Source: CAD feature listing. Evaluate the final solid. Frame: model axes, mm. A direction names the side the tool comes from. Give positions to 0.01 mm unless a question says otherwise; leave off trailing zeros. Write each loop counter-clockwise with the first axis right and the second up, starting at its lowest first coordinate (ties: lowest second). Pieces come first, ordered by that corner, then holes. Notation, with made-up numbers: (17, 82.25) -> (75, 82.25) arc R29 ccw to (75, 114.25) -> close; hole circle Ø9 at (-8.5, -15.5). An arc over 180 degrees is marked (long way). Write item = value, one per line.
from build123d import *

# Parameters (mm, degrees)
BOSS_EXTRUDE1_DEPTH = 3.5814
SKETCH2_W           = 30
SKETCH2_H           = 4
BOSS_EXTRUDE2_DEPTH = 10
SKETCH3_R           = 1.5
CUT_EXTRUDE1_DEPTH  = 4


with BuildPart() as part:
    # Sketch1 → Boss-Extrude1 (new body)
    with BuildSketch(Plane(origin=(0, 0, 0), x_dir=(1, 0, 0), z_dir=(0, 1, 0))):
        Polygon((-15, -10.05), (15, -10.05), (15, -2.05), (1.7907, -2.05), (1.7907, 2.05), (9.398, 2.05), (1.7907, 7.13), (-1.7907, 7.13), (-9.398, 2.05), (-1.7907, 2.05), (-1.7907, -2.05), (-15, -2.05), align=None)
    extrude(amount=BOSS_EXTRUDE1_DEPTH)

    # Sketch2 → Boss-Extrude2 (add)
    with BuildSketch(Plane(origin=(0, 3.5814, 0), x_dir=(1, 0, 0), z_dir=(0, 1, 0))):
        with Locations((0, -8.05)):
            Rectangle(SKETCH2_W, SKETCH2_H)
    extrude(amount=BOSS_EXTRUDE2_DEPTH)

    # Sketch3 → Cut-Extrude1 (cut)
    with BuildSketch(Plane.XY.offset(10.05)):
        with Locations((-11.65, 6.7907)):
            Circle(SKETCH3_R)
        with Locations((11.65, 6.7907)):
            Circle(SKETCH3_R)
    extrude(amount=-CUT_EXTRUDE1_DEPTH, mode=Mode.SUBTRACT)


solid = part.part
1) Contact query for flat-ended pins moving along their axis: pin 1 (1 mm diameter, centred on x = 10, y = 5, fed in from -Z); pin 2 (1.8 mm diameter, centred on x = -9.5, y = 2, fed in from -Z); pin 3 (10 mm diameter, centred on x = 11, z = -4.5, fed in from +Y). Output: stop coordinate, or through.
Computed:
pin_1 = 6.05
pin_2 = -2.58
pin_3 = 3.58
2) Cut plane B-B (y = 7.25). Return the cut outline in (x, z).
Computed:
outline = (-15, 6.05) -> (-13.08, 6.05) -> (-13.08, 10.05) -> (-15, 10.05) -> close; (-10.22, 6.05) -> (10.22, 6.05) -> (10.22, 10.05) -> (-10.22, 10.05) -> close; (13.08, 6.05) -> (15, 6.05) -> (15, 10.05) -> (13.08, 10.05) -> close
3) Cut plane D-D (z = 9.25). Return the cut outline in (x, y).
Computed:
outline = (-15, 0) -> (15, 0) -> (15, 13.58) -> (-15, 13.58) -> close; hole circle Ø3 at (-11.65, 6.79); hole circle Ø3 at (11.65, 6.79)
4) Cut plane C-C (y = 2.5). Return the cut outline in (x, z), then the cut area to 3 significant figures.
Computed:
outline = (-15, 2.05) -> (-1.79, 2.05) -> (-1.79, -2.05) -> (-9.4, -2.05) -> (-1.79, -7.13) -> (1.79, -7.13) -> (9.4, -2.05) -> (1.79, -2.05) -> (1.79, 2.05) -> (15, 2.05) -> (15, 10.05) -> (-15, 10.05) -> close
area = 312 mm²
5) Cut plane A-A (x = -11.65). Return the cut outline in (y, z), then the cut area to 3 significant figures.
Computed:
outline = (0, 2.05) -> (3.58, 2.05) -> (3.58, 6.05) -> (5.29, 6.05) -> (5.29, 10.05) -> (0, 10.05) -> close; (8.29, 6.05) -> (13.58, 6.05) -> (13.58, 10.05) -> (8.29, 10.05) -> close
area = 56.7 mm²
6) Draft query along X for faces 1 (the flat face through (15, 5, 7)), 2 (the cylindrical face through (-10.96, 5.46, 8.08)), 3 (the flat face through (-1.791, 2, 0)), 4 (the flat face through (0, 7, 10.05)). Return one class per face: pulls with the +X half, pulls with the -X half, needs draft (parallel to the pull), parting line crosses it, or undercut.
Computed:
face_1 = pulls with the +X half
face_2 = undercut
face_3 = pulls with the -X half
face_4 = needs draft
7) Access query for faces 5 (the cylindrical face through (10.15, 6.86, 8.08)), 6 (the flat face through (-6, 2, -2.05)), 7 (the flat face through (0, 3.581, 1)), 8 (the flat face through (8, 2, 2.05)). Directions: +Z, -Z, +X, -X, +Y, -Y. A direction counts if a zero-diameter tool reaches every point of the face in a straight line with its end or side. Return the directions, or none.
Computed:
face_5 = +Z, -Z
face_6 = -X, +Y, -Y
face_7 = -Z, +X, -X, +Y
face_8 = +X, +Y, -Y
8) Material intervals for L1, parallel to Y at x = -11.65, z = 8.1; L2, parallel to Z at x = -3.5, y = 4; L3, parallel to Y at x = 7.75, z = -2.25, sorted ascending.
Computed:
L1 = 0 to 5.29, 8.29 to 13.58
L2 = 6.05 to 10.05
L3 = 0 to 3.58
